The drawing under review shows one solid part. Ordinate dimensions are in mm from its lowest x, y, z. A direction names the side the tool comes from. Give positions to 0.01 mm unless a question says otherwise; leave off trailing zeros. Order: outer loops, then holes, each group sorted by start corner. A loop starts at its lowest first (then second) coordinate and runs counter-clockwise, first axis right, second up. Notation, with made-up numbers: (84, -2.75) -> (129, -2.75) arc R11 ccw to (129, 18.25) -> close; hole circle Ø5 at (52, 53.5). An arc over 180 degrees is marked (long way). One line per item, written item: value.
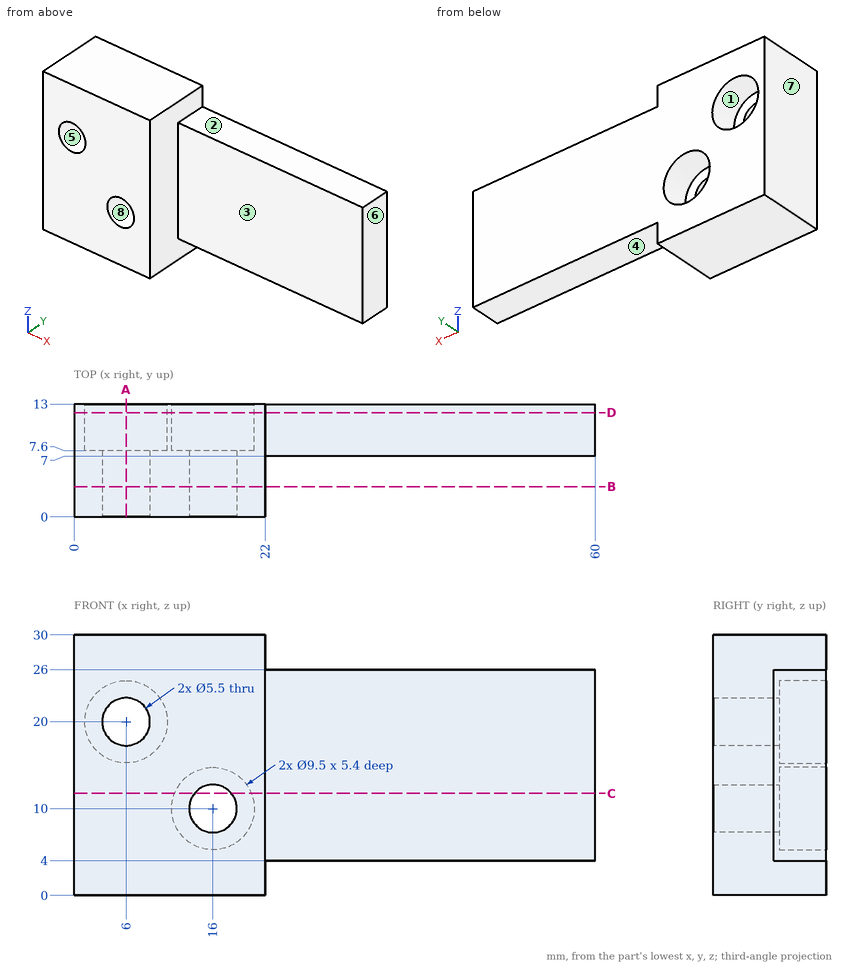
Item 1: Machinability: for the marked faces 1, 2, 3 and 4, which of the approach directions +Z, -Z, +X, -X, +Y, -Y give a long, thin tool a straight path to every point of the face, cutting with its end or side? Answer none if there is none.
Returned:
face 1: +Y
face 2: +Z, +X, +Y, -Y
face 3: +Z, -Z, +X, -Y
face 4: -Z, +X, +Y, -Y
Item 2: Add section D-D on y = 12. Give the boundary of the cut face in (x, z).
Returned:
outline: (0, 0) -> (22, 0) -> (22, 4) -> (60, 4) -> (60, 26) -> (22, 26) -> (22, 30) -> (0, 30) -> close; hole circle Ø9.5 at (6, 20); hole circle Ø9.5 at (16, 10)
Item 3: Add section B-B on y = 3.5. Give the boundary of the cut face in (x, z), plus the area to 3 significant figures.
Returned:
outline: (0, 0) -> (22, 0) -> (22, 30) -> (0, 30) -> close; hole circle Ø5.5 at (6, 20); hole circle Ø5.5 at (16, 10)
area: 612 mm²
Item 4: Add section C-C on z = 11.75. Give the boundary of the cut face in (x, y).
Returned:
outline: (0, 0) -> (13.88, 0) -> (13.88, 7.6) -> (11.58, 7.6) -> (11.58, 13) -> (0, 13) -> close; (18.12, 0) -> (22, 0) -> (22, 7) -> (60, 7) -> (60, 13) -> (20.42, 13) -> (20.42, 7.6) -> (18.12, 7.6) -> close
Item 5: To check wall thickness, follow line 1 along Z through (x, y) = (16, 5.75); line 2 along Z through (x, y) = (48.5, 11.5); line 3 along X through (y, z) = (1, 16.5). State the ranges of each line that lie inside material, in increasing order. Write a range as from..to.
Returned:
line 1: 0..7.25, 12.75..30
line 2: 4..26
line 3: 0..22
Item 6: Draft analysis for pull direction X (two halves, no side actions). For the marked faces 5, 6, 7 and 8, state which applies: pulls with the +X half, pulls with the -X half, needs draft (parallel to the pull), parting line crosses it, or undercut.
Returned:
face 5: undercut
face 6: pulls with the +X half
face 7: pulls with the -X half
face 8: undercut
Item 7: Clearance check with flat-ended pins moving along their axes: P1, Ø7, axis at x = 6, z = 20, coming from the +Y side; P2, Ø12.5, axis at x = 16, z = 10, coming from the +Y side; P3, Ø11, axis at x = 42, z = 11, coming from the -Y side; P4, Ø6.5, axis at x = 49.5, y = 10.5, coming from the -Z side. State where each tip first meets the part, or that it passes through.
Returned:
P1: y = 7.6
P2: y = 13
P3: y = 7
P4: z = 4
Item 8: Add section A-A on x = 6. Give the boundary of the cut face in (y, z).
Returned:
outline: (0, 0) -> (13, 0) -> (13, 15.25) -> (7.6, 15.25) -> (7.6, 17.25) -> (0, 17.25) -> close; (0, 22.75) -> (7.6, 22.75) -> (7.6, 24.75) -> (13, 24.75) -> (13, 30) -> (0, 30) -> close
